```python
from build123d import *

# Parameters (mm, degrees)
F0_R     = 11.25
F1_DEPTH = 1
F2_W     = 5
F2_H     = 11.54
F3_DEPTH = 12
F4_W     = 5
F4_H     = 12
F5_DEPTH = 10
F7_DEPTH = 20


with BuildPart() as f1:
    # F0 (on Top) → F1 (new body)
    with BuildSketch(Plane.XY):
        Circle(F0_R)
    extrude(amount=F1_DEPTH)

    # F2 (on face) → F3 (join)
    with BuildSketch(Plane.XY.offset(1)):
        Rectangle(F2_W, F2_H)
    extrude(amount=F3_DEPTH)

    # F4 (on Top) → F5 (join)
    with BuildSketch(Plane.XY):
        Rectangle(F4_W, F4_H)
    extrude(amount=-F5_DEPTH)

    # F6 (on face) → F7 (join)
    with BuildSketch(Plane.XY.offset(13)):
        with BuildLine():
            Line((2.5, -5.178079), (2.5, 5.178079))
            ThreePointArc((2.5, 5.178079), (0, 5.75), (-2.5, 5.178079))
            Line((-2.5, 5.178079), (-2.5, -5.178079))
            ThreePointArc((-2.5, -5.178079), (0, -5.75), (2.5, -5.178079))
        make_face()
        with BuildLine():
            Line((-2.5, -5.178079), (-2.5, 5.178079))
            ThreePointArc((-2.5, 5.178079), (-5.75, 0), (-2.5, -5.178079))
        make_face()
        with BuildLine():
            ThreePointArc((2.5, -5.178079), (4.87019, -3.056755), (5.75, 0))
            ThreePointArc((5.75, 0), (4.87019, 3.056755), (2.5, 5.178079))
            Line((2.5, 5.178079), (2.5, -5.178079))
        make_face()
    extrude(amount=F7_DEPTH)


solid = f1.part
```
Model file for the job. Use its own axes, mm. A direction names the side the tool comes from. Give positions to 0.01 mm unless a question says otherwise; leave off trailing zeros. Write each loop counter-clockwise with the first axis right and the second up, starting at its lowest first coordinate (ties: lowest second). Pieces come first, ordered by that corner, then holes. Notation, with made-up numbers: M 41.25,3 L 68.25,3 A22 cw 68.25,33 Z; hole C 74,-0.5 d8. An arc over 180 degrees is marked long. Use a Markdown table: item, result.
1) Pull direction Z, two halves, no side cores. Call faces 1 (the flat face through (0, 0, -10)), 2 (the flat face through (0, 5.77, 7)), 3 (the flat face through (4, 0, 13)): +Z half, -Z half, draft (parallel to the pull), parting line (faces both ways), or undercut.
Responses:
| item | result |
|---|---|
| face 1 | -Z half |
| face 2 | draft |
| face 3 | undercut |
2) Tool access for faces 4 (the flat face through (-2.5, 0, 7)), 5 (the flat face through (-2.5, 0, -5)), 6 (the flat face through (0, -6, -5)), 7 (the flat face through (0, 6, -5)): list every direction of +Z, -Z, +X, -X, +Y, -Y with a clear straight run to the whole face (end or side of a thin tool).
Responses:
| item | result |
|---|---|
| face 4 | -X, +Y, -Y |
| face 5 | -Z, -X, +Y, -Y |
| face 6 | -Z, +X, -X, -Y |
| face 7 | -Z, +X, -X, +Y |
3) Cut at D-D (y = 3.25). List the corners of the cut face in (x, z).
Responses:
| item | result |
|---|---|
| outline | M -10.77,0 L -2.5,0 L -2.5,-10 L 2.5,-10 L 2.5,0 L 10.77,0 L 10.77,1 L 2.5,1 L 2.5,13 L 4.74,13 L 4.74,33 L -4.74,33 L -4.74,13 L -2.5,13 L -2.5,1 L -10.77,1 Z |
4) Pin check, flat tips, straight feed: pin 1 (12 mm diameter, centred on x = -6, z = 16.5, fed in from -Y); pin 2 (5.5 mm diameter, centred on x = 1, z = -7, fed in from +Y); pin 3 (12.5 mm diameter, centred on y = 2.5, z = 4.5, fed in from -X); pin 4 (8 mm diameter, centred on y = -3, z = -4.5, fed in from -X). Stop position of each tip, or through.
Responses:
| item | result |
|---|---|
| pin 1 | stops at y = -5.77 |
| pin 2 | stops at y = 6 |
| pin 3 | stops at x = -11.25 |
| pin 4 | stops at x = -2.5 |
5) Cut at B-B (x = -3.25). List the corners of the cut face in (y, z), and give its area (3 significant figures).
Responses:
| item | result |
|---|---|
| outline | M -10.77,0 L 10.77,0 L 10.77,1 L -10.77,1 Z; M -4.74,13 L 4.74,13 L 4.74,33 L -4.74,33 Z |
| area | 211 mm2 |
6) Cut at C-C (z = 22). List the corners of the cut face in (x, y), and give its area (3 significant figures).
Responses:
| item | result |
|---|---|
| outline | M -2.5,-5.18 A5.75 ccw 2.5,-5.18 A5.75 ccw 2.5,5.18 A5.75 ccw -2.5,5.18 A5.75 ccw Z |
| area | 104 mm2 |
7) Drill centre lines: line 1 (Z direction, x = 3, y = 3.25); line 2 (X direction, y = 1.75, z = -4.5); line 3 (Z direction, x = -7.5, y = 4.75). Where is each one in solid material? Low to high. Write a range as from..to.
Responses:
| item | result |
|---|---|
| line 1 | z = 0..1, 13..33 |
| line 2 | x = -2.5..2.5 |
| line 3 | z = 0..1 |
